```python
from build123d import *

# Parameters (mm, degrees)
SKETCH_1_W          = 160
SKETCH_1_H          = 170
EXTRUDE_1_DEPTH     = 3
SKETCH_2_R          = 1.6
CUT_EXTRUDE_1_DEPTH = 13
SKETCH_3_R          = 6
CUT_EXTRUDE_2_DEPTH = 13
SKETCH_4_W          = 25
SKETCH_4_H          = 15
CUT_EXTRUDE_3_DEPTH = 13


with BuildPart() as part:
    # 草图1 → 凸台-拉伸1 (new body)
    with BuildSketch(Plane.XY):
        with Locations((35.416666667, -46.25)):
            Rectangle(SKETCH_1_W, SKETCH_1_H)
    extrude(amount=EXTRUDE_1_DEPTH)

    # 草图2 → 切除-拉伸1 (cut)
    with BuildSketch(Plane.XY.offset(3)):
        with Locations((-36.583333333, 30.75)):
            Circle(SKETCH_2_R)
        with Locations((107.416666667, 30.75)):
            Circle(SKETCH_2_R)
        with Locations((107.416666667, -123.25)):
            Circle(SKETCH_2_R)
        with Locations((-36.583333333, -123.25)):
            Circle(SKETCH_2_R)
    extrude(amount=-CUT_EXTRUDE_1_DEPTH, mode=Mode.SUBTRACT)

    # 草图3 → 切除-拉伸2 (cut)
    with BuildSketch(Plane.XY.offset(3)):
        with Locations((80.416666667, 3.75)):
            Circle(SKETCH_3_R)
    extrude(amount=-CUT_EXTRUDE_2_DEPTH, mode=Mode.SUBTRACT)

    # 草图4 → 切除-拉伸3 (cut)
    with BuildSketch(Plane.XY.offset(3)):
        with Locations((67.916666667, -98.75)):
            Rectangle(SKETCH_4_W, SKETCH_4_H)
    extrude(amount=-CUT_EXTRUDE_3_DEPTH, mode=Mode.SUBTRACT)


solid = part.part
```
Verification items for the finished model (mm, model axes). Give positions to 0.01 mm unless a question says otherwise; leave off trailing zeros. Order: outer loops, then holes, each group sorted by start corner. A loop starts at its lowest first (then second) coordinate and runs counter-clockwise, first axis right, second up. Notation, with made-up numbers: (-29, -9) -> (-11, -9) arc R15 cw to (-11, 10) -> close; hole circle Ø1 at (-29.5, -14). An arc over 180 degrees is marked (long way). One line per item, written item: value.
(1) Scan lines: line 1 along X through (y, z) = (-98.5, 1.45); line 2 along X through (y, z) = (-123.25, 1.3); line 3 along Y through (x, z) = (68.5, 2.35). Record each from-to range of solid material in increasing order. Write a range as [from, to].
Final values:
line 1: [-44.58, 55.42], [80.42, 115.42]
line 2: [-44.58, -38.18], [-34.98, 105.82], [109.02, 115.42]
line 3: [-131.25, -106.25], [-91.25, 38.75]
(2) Draft check along Y on faces 1 (the face through (86.14, 5.55, 1.52)), 2 (the face through (34, -45, 0)). Enter one of: pulls with the +Y half, pulls with the -Y half, needs draft (parallel to the pull), parting line crosses it, or undercut.
Final values:
face 1: undercut
face 2: needs draft
(3) Sectioned sample at A-A on y = 3.75. Record the cut outline in (x, z).
Final values:
outline: (-44.58, 0) -> (74.42, 0) -> (74.42, 3) -> (-44.58, 3) -> close; (86.42, 0) -> (115.42, 0) -> (115.42, 3) -> (86.42, 3) -> close
(4) Sectioned sample at B-B on z = 2.35. Record the cut outline in (x, y), then the cut area to 3 significant figures.
Final values:
outline: (-44.58, -131.25) -> (115.42, -131.25) -> (115.42, 38.75) -> (-44.58, 38.75) -> close; hole circle Ø3.2 at (-36.58, -123.25); hole circle Ø3.2 at (-36.58, 30.75); hole (55.42, -106.25) -> (80.42, -106.25) -> (80.42, -91.25) -> (55.42, -91.25) -> close; hole circle Ø12 at (80.42, 3.75); hole circle Ø3.2 at (107.42, -123.25); hole circle Ø3.2 at (107.42, 30.75)
area: 26,700 mm^2
